```python
from build123d import *

# Parameters (mm, degrees)
SKETCH_2_W          = 238.179152398
SKETCH_2_H          = 131.442897672
SKETCH_2_R          = 2
EXTRUDE_1_DEPTH     = 5
CUT_EXTRUDE_1_DEPTH = 1


with BuildPart() as part:
    # Sketch 2 → Extrude 1 (new body)
    with BuildSketch(Plane.XY):
        Rectangle(SKETCH_2_W, SKETCH_2_H)
        with BuildLine():
            Line((69, 57), (-69, 57))
            ThreePointArc((-69, 57), (-84.556349186, 50.556349186), (-91, 35))
            Line((-91, 35), (-91, -35))
            ThreePointArc((-91, -35), (-84.556349186, -50.556349186), (-69, -57))
            Line((-69, -57), (69, -57))
            ThreePointArc((69, -57), (84.556349186, -50.556349186), (91, -35))
            Line((91, -35), (91, 35))
            ThreePointArc((91, 35), (84.556349186, 50.556349186), (69, 57))
        make_face(mode=Mode.SUBTRACT)
        with BuildLine():
            ThreePointArc((69, 57), (84.556349186, 50.556349186), (91, 35))
            Line((91, 35), (91, -35))
            ThreePointArc((91, -35), (84.556349186, -50.556349186), (69, -57))
            Line((69, -57), (-69, -57))
            ThreePointArc((-69, -57), (-84.556349186, -50.556349186), (-91, -35))
            Line((-91, -35), (-91, 35))
            ThreePointArc((-91, 35), (-84.556349186, 50.556349186), (-69, 57))
            Line((-69, 57), (69, 57))
        make_face()
        with BuildLine():
            Line((69, 55), (-69, 55))
            ThreePointArc((-69, 55), (-83.142135624, 49.142135624), (-89, 35))
            Line((-89, 35), (-89, -35))
            ThreePointArc((-89, -35), (-83.142135624, -49.142135624), (-69, -55))
            Line((-69, -55), (69, -55))
            ThreePointArc((69, -55), (83.142135624, -49.142135624), (89, -35))
            Line((89, -35), (89, 35))
            ThreePointArc((89, 35), (83.142135624, 49.142135624), (69, 55))
        make_face(mode=Mode.SUBTRACT)
        with BuildLine():
            ThreePointArc((69, 55), (83.142135624, 49.142135624), (89, 35))
            Line((89, 35), (89, -35))
            ThreePointArc((89, -35), (83.142135624, -49.142135624), (69, -55))
            Line((69, -55), (-69, -55))
            ThreePointArc((-69, -55), (-83.142135624, -49.142135624), (-89, -35))
            Line((-89, -35), (-89, 35))
            ThreePointArc((-89, 35), (-83.142135624, 49.142135624), (-69, 55))
            Line((-69, 55), (69, 55))
        make_face()
        Polygon((-87, -32), (-66, -53), (66, -53), (87, -32), (87, 32), (66, 53), (-66, 53), (-87, 32), align=None, mode=Mode.SUBTRACT)
        Polygon((-87, 32), (-87, -32), (-66, -53), (66, -53), (87, -32), (87, 32), (66, 53), (-66, 53), align=None)
        with Locations((79, -32)):
            Circle(SKETCH_2_R, mode=Mode.SUBTRACT)
        with Locations((0, -48)):
            Circle(SKETCH_2_R, mode=Mode.SUBTRACT)
        with Locations((63, 45.5)):
            Circle(SKETCH_2_R, mode=Mode.SUBTRACT)
        with Locations((-63, 45.5)):
            Circle(SKETCH_2_R, mode=Mode.SUBTRACT)
        with Locations((-42.5, -5)):
            Circle(SKETCH_2_R, mode=Mode.SUBTRACT)
        with Locations((-69.5, -5)):
            Circle(SKETCH_2_R, mode=Mode.SUBTRACT)
        with Locations((-79, -32)):
            Circle(SKETCH_2_R, mode=Mode.SUBTRACT)
        with Locations((-13.5, -5)):
            Circle(SKETCH_2_R, mode=Mode.SUBTRACT)
        with Locations((13.5, -5)):
            Circle(SKETCH_2_R, mode=Mode.SUBTRACT)
        with Locations((28, -5)):
            Circle(SKETCH_2_R, mode=Mode.SUBTRACT)
        with Locations((42.5, -5)):
            Circle(SKETCH_2_R, mode=Mode.SUBTRACT)
        with Locations((69.5, -5)):
            Circle(SKETCH_2_R, mode=Mode.SUBTRACT)
        with Locations((0, 45.5)):
            Circle(SKETCH_2_R, mode=Mode.SUBTRACT)
        with Locations((-28, -5)):
            Circle(SKETCH_2_R, mode=Mode.SUBTRACT)
    extrude(amount=EXTRUDE_1_DEPTH)

    # Sketch 2_3 → Cut-Extrude 1 (cut)
    with BuildSketch(Plane.XY):
        with BuildLine():
            ThreePointArc((69, 57), (84.556349186, 50.556349186), (91, 35))
            Line((91, 35), (91, -35))
            ThreePointArc((91, -35), (84.556349186, -50.556349186), (69, -57))
            Line((69, -57), (-69, -57))
            ThreePointArc((-69, -57), (-84.556349186, -50.556349186), (-91, -35))
            Line((-91, -35), (-91, 35))
            ThreePointArc((-91, 35), (-84.556349186, 50.556349186), (-69, 57))
            Line((-69, 57), (69, 57))
        make_face()
        with BuildLine():
            Line((69, 55), (-69, 55))
            ThreePointArc((-69, 55), (-83.142135624, 49.142135624), (-89, 35))
            Line((-89, 35), (-89, -35))
            ThreePointArc((-89, -35), (-83.142135624, -49.142135624), (-69, -55))
            Line((-69, -55), (69, -55))
            ThreePointArc((69, -55), (83.142135624, -49.142135624), (89, -35))
            Line((89, -35), (89, 35))
            ThreePointArc((89, 35), (83.142135624, 49.142135624), (69, 55))
        make_face(mode=Mode.SUBTRACT)
    extrude(amount=CUT_EXTRUDE_1_DEPTH, mode=Mode.SUBTRACT)


solid = part.part
```
Input: part model. Units: mm. Frame: model coordinates. A direction names the side the tool comes from. Coordinates: 2 decimals unless noted, no trailing zeros. Put each result on its own line as item: value. Start each with the question number.
1) Reachability of faces 5 (the face through (-83.297, -48.986, 0.493)), 6 (the face through (-2, 65.721, 2)) from +Z, -Z, +X, -X, +Y, -Y: full face, straight path, thin tool, end or side. Return the list, or none.
2) Contact query for a flat-ended pin moving along its axis: pin 1 (3 mm diameter, centred on x = 28, y = -5, fed in from -Z). Output: stop coordinate, or through.
3) Mould query, pull axis X, two halves, no side actions, for faces 1 (the face through (-119.09, -1, 2)), 2 (the face through (-84.73, 50.38, 0.49)), 3 (the face through (119.09, -1, 2)), 4 (the face through (-1, 1, 0)). Classes: pulls with the +X half, pulls with the -X half, needs draft (parallel to the pull), parting line crosses it, or undercut.
4) Ray query, L1, parallel to Y at x = 5.5, z = 0.65; L2, parallel to Y at x = 28, z = 1.5; L3, parallel to Y at x = -63, z = 3.3. Return the intervals inside material, ascending.
Resolved:
1. face 5: -Z
1. face 6: +Z, -Z, +X, -X, +Y
2. pin 1: passes through
3. face 1: pulls with the -X half
3. face 2: undercut
3. face 3: pulls with the +X half
3. face 4: needs draft
4. L1: y = -65.72 to -57, -55 to 55, 57 to 65.72
4. L2: y = -65.72 to -7, -3 to 65.72
4. L3: y = -65.72 to 43.5, 47.5 to 65.72
